Part model, mm, in its own coordinate system. Face numbers are marked on the shaded views. A direction names the side the tool comes from. Round coordinates to 2 decimals unless told otherwise and drop trailing zeros. Write each loop counter-clockwise with the first axis right and the second up, starting at its lowest first coordinate (ties: lowest second). Pieces come first, ordered by that corner, then holes.
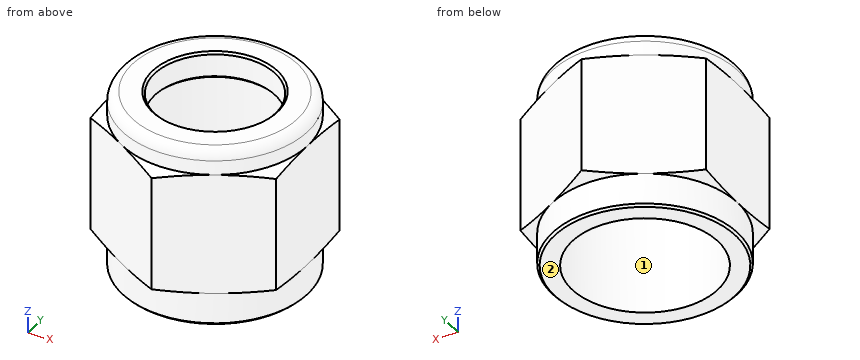
```python
from build123d import *

# Parameters (mm, degrees)
BOSS_EXTRUDE1_DEPTH = 21.5646
FILLET1_R           = 1.1938
CHAMFER1_SIZE       = 0.254
CHAMFER2_SIZE       = 0.254


with BuildPart() as part:
    # Sketch1 → Boss-Extrude1 (new body)
    with BuildSketch(Plane.XY):
        Polygon((0, 12.831609733), (-11.1125, 6.415804866), (-11.1125, -6.415804866), (0, -12.831609733), (11.1125, -6.415804866), (11.1125, 6.415804866), align=None)
    extrude(amount=BOSS_EXTRUDE1_DEPTH)

    # Sketch2 → Cut-Revolve1 (revolve, cut)
    with BuildSketch(Plane(origin=(0, 0, 0), x_dir=(0, 0, -1), z_dir=(1, 0, 0))):
        Polygon((-21.5646, 14.550719465), (-21.5646, 11.1125), (-18.6436, 11.1125), (-18.182965935, 12.831609733), (-4.423034065, 12.831609733), (-3.9624, 11.1125), (0, 11.1125), (0, 14.550719465), align=None)
        with BuildLine():
            Line((-21.5646, 7.239), (-21.5646, 0))
            Line((-21.5646, 0), (0, 0))
            Line((0, 0), (0, 8.751666378))
            Line((0, 8.751666378), (-18.1102, 8.751666378))
            ThreePointArc((-18.1102, 8.751666378), (-18.289805122, 8.6772715), (-18.3642, 8.497666378))
            Line((-18.3642, 8.497666378), (-18.3642, 7.239))
            Line((-18.3642, 7.239), (-21.5646, 7.239))
        make_face()
    revolve(axis=Axis((0, 0, 0), (0, 0, 1)), mode=Mode.SUBTRACT)

    # Fillet1
    fillet1_edges = [part.edges().sort_by_distance(p)[0] for p in [
        (0, -11.1125, 21.5646),
    ]]
    fillet(fillet1_edges, radius=FILLET1_R)

    # Chamfer1
    chamfer1_edges = [part.edges().sort_by_distance(p)[0] for p in [
        (0, -11.1125, 0),
    ]]
    chamfer(chamfer1_edges, length=CHAMFER1_SIZE)

    # Chamfer2
    chamfer2_edges = [part.edges().sort_by_distance(p)[0] for p in [
        (0, -7.239, 21.5646),
        (0, -7.239, 18.3642),
    ]]
    chamfer(chamfer2_edges, length=CHAMFER2_SIZE)


solid = part.part
```
Q1. Cut at A-A on z = 13.25. Write the cut outline in (x, y), plus the area to 3 significant figures.
Values follow:
outline: (-11.11, -6.42) - (0, -12.83) - (11.11, -6.42) - (11.11, 6.42) - (0, 12.83) - (-11.11, 6.42) - close; hole circle Ø17.5 at (0, 0)
area: 187 mm2
Q2. Cut at B-B on z = 1.75. Write the cut outline in (x, y) (1 decimal).
Values follow:
outline: circle Ø22.2 at (0, 0); hole circle Ø17.5 at (0, 0)
Q3. Wall check: L1, parallel to Y at x = 0, z = 19.7; L2, parallel to X at y = -4, z = 12.75. Give the ranges that are in metal, low to high.
Values follow:
L1: y = -11.11 to -7.24, 7.24 to 11.11
L2: x = -11.11 to -7.78, 7.78 to 11.11
Q4. Drop flat-ended pins along their axis: pin 1 (6 mm diameter, centred on x = 5.5, z = 7.5, fed in from -Y); pin 2 (5 mm diameter, centred on x = 5.5, z = 12, fed in from +Y). Give the stop position or say it passes through.
Values follow:
pin 1: stops at y = -11.39
pin 2: stops at y = 11.1
Q5. Which spindle directions (+Z, -Z, +X, -X, +Y, -Y) get a long thin tool onto all of the face, cutting with end or side? Do the marked faces 1 and 2. Say none if no direction does.
Values follow:
face 1: -Z
face 2: -Z, +X, -X, +Y, -Y
